For this review, take the finished solid that the model builds, in its own axes (mm). A direction names the side the tool comes from. Give positions to 0.01 mm unless a question says otherwise; leave off trailing zeros. Write each loop counter-clockwise with the first axis right and the second up, starting at its lowest first coordinate (ties: lowest second). Pieces come first, ordered by that corner, then holes.
Q1. We need section C-C (z = 0.5). Write out the cut boundary in (x, y).
Q2. Machinability: for faces 1 (the flat face through (5.5, -46.8, 2.45)), 2 (the flat face through (4, -30, 0)), which of the approach directions +Z, -Z, +X, -X, +Y, -Y give a long, thin tool a straight path to every point of the face, cutting with its end or side? Answer none if there is none.
Q3. Mouldability with a two-part tool opening along Y and no side actions: class faces 3 (the flat face through (0, -31, 2)), 4 (the flat face through (4, -60.8, 2)), 5 (the cylindrical face through (4.575, -19.664, 1.208)) as released by +Y, released by -Y, zero draft, split by the parting line, or undercut.
Q4. For line 1 (Y direction, x = 4.25, z = 0.75); line 2 (Y direction, x = 4.25, z = 3.2); line 3 (Z direction, x = 2.75, y = -45), list the stretches that pass through material, from the lowest coordinate up.
Q5. Insertion check: P1, Ø3, axis at x = 5, y = -46, coming from the +Z side; P2, Ø2.5, axis at x = 4.25, y = -18.2, coming from the -Z side. Each pin has a flat end and moves straight along its axis. Give the tip position at first contact, or say it passes through.
Q6. We need section A-A (y = -45.6). Write out the cut boundary in (x, z), then the cut area to 3 significant figures.
Q7. We need section B-B (x = 4.25). Write out the cut boundary in (y, z).
Q8. We need section D-D (z = 3.65). Write out the cut boundary in (x, y), then the cut area to 3 significant figures.
```python
from build123d import *

# Parameters (mm, degrees)
SKETCH1_W                 = 8.5
SKETCH1_H                 = 60.8
BOSS_EXTRUDE1_DEPTH       = 4.65
F_3_0MM_DOWEL_HOLE1_D     = 3
F_3_0MM_DOWEL_HOLE1_DEPTH = 5
F_3_0MM_DOWEL_HOLE1_TIP   = 0.901290929
SKETCH6_R                 = 2.85
CUT_EXTRUDE1_DEPTH        = 2.2


with BuildPart() as part:
    # Sketch1 → Boss-Extrude1 (new body)
    with BuildSketch(Plane.XY):
        with Locations((4.25, -30.4)):
            Rectangle(SKETCH1_W, SKETCH1_H)
    extrude(amount=BOSS_EXTRUDE1_DEPTH)

    # Ø3.0mm Dowel Hole1
    with Locations(Plane.XY.offset(4.65)):
        with Locations((4.25, -18.2), (4.25, -45.6)):
            Hole(F_3_0MM_DOWEL_HOLE1_D / 2, depth=F_3_0MM_DOWEL_HOLE1_DEPTH)
            with Locations((0, 0, -(F_3_0MM_DOWEL_HOLE1_DEPTH + F_3_0MM_DOWEL_HOLE1_TIP / 2))):  # 118° drill point
                Cone(0, F_3_0MM_DOWEL_HOLE1_D / 2, F_3_0MM_DOWEL_HOLE1_TIP, mode=Mode.SUBTRACT)

    # Sketch6 → Cut-Extrude1 (cut)
    with BuildSketch(Plane.XY.offset(4.65)):
        with Locations((4.25, -18.2)):
            Circle(SKETCH6_R)
        with Locations((4.25, -45.6)):
            Circle(SKETCH6_R)
    extrude(amount=-CUT_EXTRUDE1_DEPTH, mode=Mode.SUBTRACT)


solid = part.part
```
Computed:
1. outline: (0, -60.8) - (8.5, -60.8) - (8.5, 0) - (0, 0) - close; hole circle Ø3 at (4.25, -45.6); hole circle Ø3 at (4.25, -18.2)
2. face 1: +Z
2. face 2: -Z, +X, -X, +Y, -Y
3. face 3: zero draft
3. face 4: released by -Y
3. face 5: undercut
4. line 1: y = -60.8 to -47.1, -44.1 to -19.7, -16.7 to 0
4. line 2: y = -60.8 to -48.45, -42.75 to -21.05, -15.35 to 0
4. line 3: z = 0 to 2.45
5. P1: stops at z = 2.45
5. P2: passes through
6. outline: (0, 0) - (2.75, 0) - (2.75, 2.45) - (1.4, 2.45) - (1.4, 4.65) - (0, 4.65) - close; (5.75, 0) - (8.5, 0) - (8.5, 4.65) - (7.1, 4.65) - (7.1, 2.45) - (5.75, 2.45) - close
6. area: 19.6 mm2
7. outline: (-60.8, 0) - (-47.1, 0) - (-47.1, 2.45) - (-48.45, 2.45) - (-48.45, 4.65) - (-60.8, 4.65) - close; (-44.1, 0) - (-19.7, 0) - (-19.7, 2.45) - (-21.05, 2.45) - (-21.05, 4.65) - (-42.75, 4.65) - (-42.75, 2.45) - (-44.1, 2.45) - close; (-16.7, 0) - (0, 0) - (0, 4.65) - (-15.35, 4.65) - (-15.35, 2.45) - (-16.7, 2.45) - close
8. outline: (0, -60.8) - (8.5, -60.8) - (8.5, 0) - (0, 0) - close; hole circle Ø5.7 at (4.25, -45.6); hole circle Ø5.7 at (4.25, -18.2)
8. area: 466 mm2
